Autodesk Inventor part; units mm, degrees
ref_plane "YZ Plane" through (0, 0, 0) normal (1, 0, 0) x (0, 1, 0)
ref_plane "XZ Plane" through (0, 0, 0) normal (0, 1, 0) x (-1, 0, 0)
ref_plane "XY Plane" through (0, 0, 0) normal (0, 0, 1) x (1, 0, 0)
sketch "Sketch1" plane through (0, 0, 0) normal (0, 0, 1) x (1, 0, 0)
  arc A0 (-3.1, 0) -> (3.1, 0) centre (0, 0) ccw
  arc A1 (-5.5, 0) -> (5.5, 0) centre (0, 0) ccw
  line L0 (-3.1, 0) -> (-5.5, 0)
  line L1 (-5.5, 0) -> (-5.5, 5.5)
  line L2 (-5.5, 5.5) -> (-3.1, 5.5)
  line L3 (-3.1, 5.5) -> (-3.1, 0)
  line L4 (3.1, 0) -> (5.5, 0)
  line L5 (5.5, 0) -> (5.5, 5.5)
  line L6 (5.5, 5.5) -> (3.1, 5.5)
  line L7 (3.1, 5.5) -> (3.1, 0)
  line L8 (-5.5, 0) -> (-5.5, 5.5)
  line L9 (-5.5, 5.5) -> (-12.5, 5.5)
  line L10 (-12.5, 5.5) -> (-12.5, 0)
  line L11 (-12.5, 0) -> (-5.5, 0)
  line L12 (5.5, 0) -> (5.5, 5.5)
  line L13 (5.5, 5.5) -> (12.5, 5.5)
  line L14 (12.5, 5.5) -> (12.5, 0)
  line L15 (12.5, 0) -> (5.5, 0)
  line L16 (12.5, 0) -> (12.5, -5.5)
  line L17 (12.5, -5.5) -> (-12.5, -5.5)
  line L18 (-12.5, -5.5) -> (-12.5, 0)
  dimension "d0" = 6.2
  dimension "d1" = 11
  dimension "d2" = 7
  dimension "d3" = 7
extrude "Extr-legs" add sketch "Sketch1" along normal blind 40 contours L11 L10 L9 L1 | L5 L13 L14 L15
extrude "Extr-base" add sketch "Sketch1" against normal blind 5 contours A0 L4 A1 L0 | L0 L1 L2 L3 | L7 L6 L5 L4 | L11 L10 L9 L1 | L5 L13 L14 L15
sketch "Sketch2" plane through (0, 0, 40) normal (0, 0, 1) x (1, 0, 0)
  circle A0 centre (0, 0) radius 2.2
  circle A1 centre (0, 0) radius 4.5
  line L0 (5.5, 0) -> (12.5, 0)
  line L1 (-12.5, 0) -> (-5.5, 0)
  line L2 (-12.5, 0) -> (-12.5, 5.5)
  line L3 (-12.5, 5.5) -> (12.5, 5.5)
  line L4 (12.5, 5.5) -> (12.5, 0)
  line L5 (12.5, 0) -> (2.2, 0)
  line L6 (-2.2, 0) -> (-12.5, 0)
  line L7 (-12.5, 0) -> (-12.5, -4.5048)
  line L8 (-12.5, -4.5048) -> (12.5, -4.5048)
  line L9 (12.5, -4.5048) -> (12.5, 0)
  line L10 (12.5, 0) -> (5.5, 0)
  line L11 (12.5, 0) -> (3.5, 0)
  line L12 (3.5, 0) -> (3.5, -4.5048)
  line L13 (3.5, -4.5048) -> (12.5, -4.5048)
  line L14 (12.5, -4.5048) -> (12.5, 0)
  line L15 (-12.5, 0) -> (-7.5, 0)
  line L16 (-7.5, 0) -> (-7.5, -4.5048)
  line L17 (-7.5, -4.5048) -> (-12.5, -4.5048)
  line L18 (-12.5, -4.5048) -> (-12.5, 0)
  dimension "d8" = 4.4
  dimension "d9" = 9
extrude "Extr-top" add sketch "Sketch2" along normal blind 5 contours L5 L12 A1 L6 A0 | A0 L6 A1 L5 | L5 A1 L12 | L6 L1 L2 L3 L4 L0 L5 A1 | A1 L12 L8 L16 L1 L6 | L5 L0 L9 L8 L12 A1 | L16 L8 L7 L1
extrude "Extrusion4" add sketch "Sketch1" against normal up to surface (5 mm away) contours A1 L17 L18 L11 | L15 L16 L17 A1
sketch "Sketch3" plane through (0, 0, 40) normal (0, 0, -1) x (-1, 0, 0)
  line L0 (-5.5, 0) -> (-12.5, 0)
  line L1 (-12.5, -4.5048) -> (-12.5, 0)
  line L2 (12.5, -4.5048) -> (-12.5, -4.5048)
  line L3 (12.5, 0) -> (12.5, -4.5048)
  line L4 (12.5, 0) -> (5.5, 0)
  line L5 (5.5, 0) -> (5.5, 5.5)
  line L6 (-5.5, 5.5) -> (5.5, 5.5)
  line L7 (-5.5, 5.5) -> (-5.5, 0)
  circle A0 centre (0, 0) radius 2.2
  line L8 (12.5, -4.5048) -> (-12.5, -4.5048)
  line L9 (-12.5, 0) -> (-5.5, 0)
  line L10 (-5.5, 0) -> (-5.5, -4.5048)
  line L11 (-5.5, -4.5048) -> (-12.5, -4.5048)
  line L12 (-12.5, -4.5048) -> (-12.5, 0)
  line L13 (12.5, 0) -> (5.5, 0)
  line L14 (5.5, 0) -> (12.5, 0)
  line L15 (12.5, 0) -> (12.5, -4.5048)
  line L16 (12.5, -4.5048) -> (5.5, -4.5048)
  line L17 (5.5, -4.5048) -> (5.5, 0)
extrude "Extrusion5" add sketch "Sketch3" along normal up to next contours L10 L2 L1 L0 | L17 L4 L3 L2
sketch "Sketch4" plane through (0, 0, 0) normal (0, 0, 1) x (1, 0, 0)
  line L0 (-12.5, -5.5) -> (12.5, -5.5)
  line L1 (-5.5, -4.5048) -> (-12.5, -4.5048)
  line L2 (-12.5, -5.5) -> (-5.5, -5.5)
  line L3 (-5.5, -5.5) -> (-5.5, -4.5048)
  line L4 (-5.5, -4.5048) -> (-12.5, -4.5048)
  line L5 (-12.5, -4.5048) -> (-12.5, -5.5)
  line L6 (12.5, -4.5048) -> (5.5, -4.5048)
  line L7 (-12.5, -5.5) -> (12.5, -5.5)
  line L8 (12.5, -4.5048) -> (5.5064, -4.5048)
  line L9 (5.5064, -4.5048) -> (5.5064, -5.5)
  line L10 (5.5064, -5.5) -> (12.5, -5.5)
  line L11 (12.5, -5.5) -> (12.5, -4.5048)
  point P0 (0, 0)
extrude "Extrusion6" add sketch "Sketch4" along normal up to surface (45 mm away)
sketch "Sketch5" plane through (0, 0, 45) normal (0, 0, 1) x (1, 0, 0)
  line L0 (-5.5, -4.5048) -> (5.5, -4.5048)
  line L1 (-12.5, -5.5) -> (12.5, -5.5)
  line L2 (-5.5, -4.5048) -> (5.516, -4.5048)
  line L3 (5.516, -4.5048) -> (5.516, -5.5)
  line L4 (5.516, -5.5) -> (-5.5, -5.5)
  line L5 (-5.5, -5.5) -> (-5.5, -4.5048)
  point P0 (0, 0)
extrude "Extrusion7" add sketch "Sketch5" against normal up to surface (5 mm away)
properties part number "cage2table-mount-M4(top)-M6(bottom)"
Design review of the part built by this model. Coordinates are the model's own, in mm. A direction names the side the tool comes from. Coordinates: 2 decimals unless noted, no trailing zeros. Order: outer loops, then holes, each group sorted by start corner. A loop starts at its lowest first (then second) coordinate and runs counter-clockwise, first axis right, second up.
Item 1: For faces 4 (the flat face through (0, 3, 45)), 5 (the flat face through (3.1, 3, -2)), 6 (the flat face through (0, 3, 40)), list the 3-axis set-ups (+Z, -Z, +X, -X, +Y, -Y) from which the entire face can be reached by the end or side of a thin tool; tool diameter is ignored.
Item 2: Take a section at B-B, the plane x = 0. Write out the cut boundary in (y, z), then the cut area to 3 significant figures.
Item 3: For line 1 (Z direction, x = -5, y = 1); line 2 (X direction, y = -2.25, z = 33.5); line 3 (X direction, y = 0, z = 42.15), list the stretches that pass through material, from the lowest coordinate up.
Item 4: Take a section at C-C, the plane x = -4. Write out the cut boundary in (y, z), then the cut area to 3 significant figures.
Item 5: The part is to be moulded in two halves that separate along X. For faces 1 (the flat face through (0, -4, 0)), 2 (the flat face through (6, 5.5, 20)), 3 (the flat face through (-12.5, 0, 20)), say which applies: pulls with the +X half, pulls with the -X half, needs draft (parallel to the pull), parting line crosses it, or undercut.
Item 6: Take a section at D-D, the plane y = 3.25. Write out the cut boundary in (x, z).
Item 7: For pin 1 Ø5.5 at (x, y) = (0, 0) entering from -Z, flat-tipped, find the tip position at first contact; note if it passes through.
The answers:
1. face 4: +Z, +X, -X, +Y, -Y
1. face 5: -Z, +Y
1. face 6: +Y, -Y
2. outline: (-5.5, -5) - (-3.1, -5) - (-3.1, 0) - (-5.5, 0) - close; (-5.5, 40) - (-2.2, 40) - (-2.2, 45) - (-5.5, 45) - close; (2.2, 40) - (5.5, 40) - (5.5, 45) - (2.2, 45) - close
2. area: 45.0 mm2
3. line 1: z = -5 to 0, 40 to 45
3. line 2: x = -12.5 to -5.5, 5.5 to 12.5
3. line 3: x = -12.5 to -2.2, 2.2 to 12.5
4. outline: (-5.5, -5) - (5.5, -5) - (5.5, 0) - (-5.5, 0) - close; (-5.5, 40) - (5.5, 40) - (5.5, 45) - (-5.5, 45) - close
4. area: 110 mm2
5. face 1: undercut
5. face 2: needs draft
5. face 3: pulls with the -X half
6. outline: (-12.5, -5) - (-3.1, -5) - (-3.1, 0) - (-5.5, 0) - (-5.5, 40) - (5.5, 40) - (5.5, 0) - (3.1, 0) - (3.1, -5) - (12.5, -5) - (12.5, 45) - (-12.5, 45) - close
7. pin 1: stops at z = 40
